Could you check a few things on this model? Use its own coordinates, in mm. A direction names the side the tool comes from. Round coordinates to 2 decimals unless told otherwise and drop trailing zeros. Loops run counter-clockwise (first coordinate to the right, second up) from the corner with the lowest first, then second, coordinate; pieces in that order, holes last. Notation, with made-up numbers: (0, -0.75) -> (55, -0.75) arc R16 cw to (55, 11.25) -> close; hole circle Ø7 at (-9.75, 4). An arc over 180 degrees is marked (long way). Write each question's results on one line, items separated by ' | '. Start each with the question number.
1) Imagine slicing it at C-C, the plane y = 37. List the corners of the cut face in (x, z) for me, plus the area to 3 significant figures.
2) Imagine slicing it at D-D, the plane x = -19.5. List the corners of the cut face in (y, z) for me, plus the area to 3 significant figures.
3) Imagine slicing it at A-A, the plane z = 1.25. List the corners of the cut face in (x, y) for me, plus the area to 3 significant figures.
4) If I drill on probe 1 along X at (y, z) = (26, 1.05); probe 2 along Y at (x, z) = (-30, 1.15); probe 3 along Y at (x, z) = (-29.5, 1.35), over which ranges is the centre line in solid material (lowest first)?
5) Imagine slicing it at B-B, the plane x = -30. List the corners of the cut face in (y, z) for me.
6) Which directions (+Z, -Z, +X, -X, +Y, -Y) give clear straight access to the entire face, cutting with the end or side of a thin tool? Please do faces 1 (the flat face through (29.56, 21.22, 0.76)), 2 (the flat face through (-30.25, 21.28, 0.76)), 3 (the cylindrical face through (-28.89, 24.99, 0.76)).
7) For P1, Ø1.8, axis at x = 29.65, y = 25.89, coming from the +Z side, with a flat end and sliding along its axis, tell me the tip position at first contact or that it passes through.
8) We'd pull the mould along Y, two halves only. Please class faces 4 (the cylindrical face through (0.1, -0.1, 0.7)), 5 (the flat face through (29.95, 13.62, 0.76)), 6 (the cylindrical face through (22.076, 48.136, 0.76)): pulls with the +Y half, pulls with the -Y half, needs draft (parallel to the pull), parting line crosses it, or undercut.
Autodesk Fusion 360 part; units mm, degrees
sketch "スケッチ1" plane through (0, 0, 0) normal (0, 0, 1) x (1, 0, 0)
  arc A0 (-42.8671, 10.2928) -> (42.0947, 10.2928) centre (-0.3862, 91.8977) ccw
  line L0 (-0.3862, 91.8977) -> (-42.8671, 10.2928) construction
  line L1 (-0.3862, 91.8977) -> (42.0947, 10.2928) construction
  line L2 (-42.8671, 10.2928) -> (-23.0119, 48.4342)
  line L3 (42.0947, 10.2928) -> (22.2395, 48.4342)
  line L4 (-23.0119, 48.4342) -> (22.2395, 48.4342)
  dimension "d1" = 92
  dimension "d2" = 55
  dimension "d3" = 43
  dimension "d4" = 43
extrude "押し出し1" add sketch "スケッチ1" along normal blind 1.5
sketch "スケッチ2" plane through (0, 0, 1.5) normal (0, 0, 1) x (-1, 0, 0)
  arc A0 (42.8671, -10.2928) -> (-42.0947, -10.2928) centre (0.3862, -91.8977) ccw
  line L0 (-42.0947, -10.2928) -> (-22.2395, -48.4342)
  line L1 (-22.2395, -48.4342) -> (23.0119, -48.4342)
  line L2 (23.0119, -48.4342) -> (42.8671, -10.2928)
  line L3 (42.8671, -10.2928) -> (34.7865, -25.8154)
  line L4 (-42.0947, -10.2928) -> (-34.0141, -25.8154)
  line L5 (34.7865, -25.8154) -> (26.6537, -17.6847)
  line L6 (26.6537, -17.6847) -> (36.8874, -7.4486)
  line L7 (36.8874, -7.4486) -> (42.8671, -10.2928)
  line L8 (34.7865, -25.8154) -> (42.8671, -10.2928)
  line L9 (-34.0141, -25.8154) -> (-26.0125, -17.5556)
  line L10 (-26.0125, -17.5556) -> (-36.1199, -7.4507)
  line L11 (-36.1199, -7.4507) -> (-42.0947, -10.2928)
  dimension "d7" = 17.5
  dimension "d8" = 17.5
  dimension "d9" = 11.5
  dimension "d10" = 11.5
extrude "押し出し2" cut sketch "スケッチ2" against normal blind 1.5 contours L2 L3 L5 L6 L7 L8
extrude "押し出し3" cut sketch "スケッチ2" against normal blind 1.5 contours L0 L4 L9 L10 L11
sketch "スケッチ3" plane through (0, 0, 1.5) normal (0, 0, 1) x (-1, 0, 0)
  line L0 (-36.1199, -7.4507) -> (-26.0125, -17.5556)
  line L1 (-26.0125, -17.5556) -> (-34.0141, -25.8154)
  line L2 (-34.0141, -25.8154) -> (-22.2395, -48.4342)
  line L3 (-22.2395, -48.4342) -> (23.0119, -48.4342)
  line L4 (23.0119, -48.4342) -> (34.7865, -25.8154)
  line L5 (34.7865, -25.8154) -> (26.6537, -17.6847)
  line L6 (26.6537, -17.6847) -> (36.8874, -7.4486)
  arc A0 (36.8874, -7.4486) -> (-36.1199, -7.4507) centre (0.3862, -91.8977) ccw
  line L7 (45.6832, -13.5395) -> (36.8874, -13.5395)
  line L8 (36.8874, -13.5395) -> (36.8874, -7.4486)
  line L9 (36.8874, -7.4486) -> (45.6832, -7.4486)
  line L10 (45.6832, -7.4486) -> (45.6832, -13.5395)
  line L11 (-36.1199, -7.4507) -> (-43.0096, -7.4507)
  line L12 (-43.0096, -7.4507) -> (-43.0096, -10.616)
  line L13 (-43.0096, -10.616) -> (-36.1199, -10.616)
  line L14 (-36.1199, -10.616) -> (-36.1199, -7.4507)
extrude "押し出し4" cut sketch "スケッチ3" against normal blind 1.5 contours L7 L8 L9 L10
extrude "押し出し5" cut sketch "スケッチ3" against normal blind 1.5 contours L11 L12 L13 L14
fillet "フィレット1" radius 2 1 edges at (-36.8874, 7.4486, 0.75)
fillet "フィレット2" radius 2 1 edges at (-34.7865, 25.8154, 0.75)
fillet "フィレット3" radius 2 1 edges at (36.1199, 7.4507, 0.75)
fillet "フィレット4" radius 2 1 edges at (22.2395, 48.4342, 0.75)
fillet "フィレット5" radius 2 1 edges at (-23.0119, 48.4342, 0.75)
fillet "フィレット6" radius 2 1 edges at (34.0141, 25.8154, 0.75)
sketch "スケッチ4" plane through (0, 0, 1.5) normal (0, 0, 1) x (-1, 0, 0)
  arc A0 (-33.0106, -24.7796) -> (-33.3482, -27.0947) centre (-31.5741, -26.1712) ccw
  line L0 (-33.3482, -27.0947) -> (-22.7999, -47.3577)
  arc A1 (-22.7999, -47.3577) -> (-21.0259, -48.4342) centre (-21.0259, -46.4342) ccw
  line L1 (-21.0259, -48.4342) -> (21.7982, -48.4342)
  arc A2 (21.7982, -48.4342) -> (23.5723, -47.3577) centre (21.7982, -46.4342) ccw
  line L2 (23.5723, -47.3577) -> (34.1092, -27.1164)
  arc A3 (34.1092, -27.1164) -> (33.7492, -24.7785) centre (32.3352, -26.1929) ccw
  line L3 (33.7492, -24.7785) -> (26.6537, -17.6847)
  line L4 (26.6537, -17.6847) -> (34.7689, -9.5676)
  arc A4 (34.7689, -9.5676) -> (34.0871, -6.2926) centre (33.3545, -8.1536) ccw
  arc A5 (34.0871, -6.2926) -> (-33.3191, -6.2943) centre (0.3862, -91.8977) ccw
  arc A6 (-33.3191, -6.2943) -> (-34.0004, -9.5696) centre (-32.5864, -8.1552) ccw
  line L5 (-34.0004, -9.5696) -> (-26.0125, -17.5556)
  line L6 (-26.0125, -17.5556) -> (-33.0106, -24.7796)
  circle A7 centre (30, -26) radius 1.5
  circle A8 centre (-29.6492, -25.8885) radius 1.5
  dimension "d31" = 3
  dimension "d32" = 3
extrude "押し出し6" cut sketch "スケッチ4" against normal blind 2 contours A8
extrude "押し出し7" cut sketch "スケッチ4" against normal blind 2 contours A7
Checked values:
1) outline: (-28.96, 0) -> (28.19, 0) -> (28.19, 1.5) -> (-28.96, 1.5) -> close | area: 85.7 mm^2
2) outline: (1.91, 0) -> (48.43, 0) -> (48.43, 1.5) -> (1.91, 1.5) -> close | area: 69.8 mm^2
3) outline: (-34.77, 9.57) arc R2 ccw to (-34.09, 6.29) arc R92 ccw to (33.32, 6.29) arc R2 ccw to (34, 9.57) -> (26.01, 17.56) -> (33.01, 24.78) arc R2 ccw to (33.35, 27.09) -> (22.8, 47.36) arc R2 ccw to (21.03, 48.43) -> (-21.8, 48.43) arc R2 ccw to (-23.57, 47.36) -> (-34.11, 27.12) arc R2 ccw to (-33.75, 24.78) -> (-26.65, 17.68) -> close; hole circle Ø3 at (-30, 26); hole circle Ø3 at (29.65, 25.89) | area: 2,780 mm^2
4) probe 1: -34.33 to -31.5, -28.5 to 28.15, 31.15 to 33.57 | probe 2: 4.79 to 14.34, 21.03 to 24.5, 27.5 to 35.01 | probe 3: 4.63 to 14.84, 20.53 to 24.59, 27.41 to 35.97
5) outline: (4.79, 0) -> (14.34, 0) -> (14.34, 1.5) -> (4.79, 1.5) -> close; (21.03, 0) -> (24.5, 0) -> (24.5, 1.5) -> (21.03, 1.5) -> close; (27.5, 0) -> (35.01, 0) -> (35.01, 1.5) -> (27.5, 1.5) -> close
6) face 1: +Z, -Z, +X | face 2: +Z, -Z, -X | face 3: +Z, -Z
7) P1: through
8) face 4: pulls with the -Y half | face 5: undercut | face 6: pulls with the +Y half
